from build123d import *

# Parameters (mm, degrees)
F0_W      = 79.172081314
F0_H      = 54.2475348338
F1_DEPTH  = 2
F2_W      = 79.172081314
F2_H      = 1.9382014871
F3_DEPTH  = 4
F4_W      = 52.3093333468
F4_H      = 4
F5_DEPTH  = 2.3
F6_W      = 76.872081314
F6_H      = 4
F7_DEPTH  = 2.1
F8_W      = 50.2093333468
F8_H      = 4
F9_DEPTH  = 2.4
F10_R     = 11.306687144
F11_DEPTH = 21
F12_R     = 9.8017826829
F13_DEPTH = 11
F14_R     = 8.8437005901
F15_DEPTH = 18


with BuildPart() as f1:
    # F0 (on Top) → F1 (new body)
    with BuildSketch(Plane.XY):
        with Locations((-27.7679827996, 36.830064375)):
            Rectangle(F0_W, F0_H)
    extrude(amount=F1_DEPTH)

    # F2 (on face) → F3 (join)
    with BuildSketch(Plane.XY.offset(2)):
        with Locations((-27.7679827996, 62.9847310483)):
            Rectangle(F2_W, F2_H)
    extrude(amount=F3_DEPTH)

    # F4 (on face) → F5 (join)
    with BuildSketch(Plane.YZ.offset(11.8180578575)):
        with Locations((35.8609636314, 4)):
            Rectangle(F4_W, F4_H)
    extrude(amount=-F5_DEPTH)

    # F6 (on face) → F7 (join)
    with BuildSketch(Plane.XZ.offset(-9.706296958)):
        with Locations((-28.9179827996, 4)):
            Rectangle(F6_W, F6_H)
    extrude(amount=-F7_DEPTH)

    # F8 (on face) → F9 (join)
    with BuildSketch(Plane(origin=(-67.3540234566, 0, 0), x_dir=(0, -1, 0), z_dir=(-1, 0, 0))):
        with Locations((-36.9109636314, 4)):
            Rectangle(F8_W, F8_H)
    extrude(amount=-F9_DEPTH)

    # F10 (on face) → F11 (join)
    with BuildSketch(Plane.XY.offset(2)):
        with Locations((-31.4333550632, 37.8074981272)):
            Circle(F10_R)
    extrude(amount=F11_DEPTH)

    # F12 (on face) → F13 (join)
    with BuildSketch(Plane.XY.offset(23)):
        with Locations((-31.4333550632, 37.8074981272)):
            Circle(F12_R)
    extrude(amount=-F13_DEPTH)

    # F14 (on face) → F15 (cut)
    with BuildSketch(Plane.XY.offset(23)):
        with Locations((-31.4333550632, 37.8074981272)):
            Circle(F14_R)
    extrude(amount=-F15_DEPTH, mode=Mode.SUBTRACT)


solid = f1.part
The model under review builds one solid part; all positions refer to its coordinate system, in mm. A direction names the side the tool comes from. Give positions to 0.01 mm unless a question says otherwise; leave off trailing zeros. Order: outer loops, then holes, each group sorted by start corner. A loop starts at its lowest first (then second) coordinate and runs counter-clockwise, first axis right, second up. Notation, with made-up numbers: M 38.5,-6 L 43.5,-6 A24 cw 43.5,11 Z; hole C -21,81 d4. An arc over 180 degrees is marked long. Answer in a Markdown table with one row per item. Add a question column.
1. To check wall thickness, follow line 1 along Y through (x, z) = (-35.5, 4.5); line 2 along X through (y, z) = (20, 4.5); line 3 along Z through (x, y) = (-25.5, 35.5). State the ranges of each line that lie inside material, in increasing order.
2. Add section D-D on x = -29. State the section outline as (y, z) points, plus the area to 3 significant figures.
3. Mouldability with a two-part tool opening along Y and no side actions: class faces 3 (the cylindrical face through (-25.35, 47.34, 12.35)), 4 (the flat face through (-28, 9.706, 3)), 5 (the flat face through (-28, 63, 6)), 6 (the flat face through (-64.954, 37, 4)) as released by +Y, released by -Y, zero draft, split by the parting line, or undercut.
4. Machinability: for faces 1 (the flat face through (11.818, 36, 3)), 2 (the flat face through (-28, 62.016, 4)), which of the approach directions +Z, -Z, +X, -X, +Y, -Y give a long, thin tool a straight path to every point of the face, cutting with its end or side? Answer none if there is none.
5. Add section B-B on x = 4. State the section outline as (y, z) points, plus the area to 3 significant figures.
6. Add section C-C on z = 16. State the section outline as (x, y) points.
7. For pin 1 Ø5 at (x, y) = (-25, 20.5) entering from +Z; pin 2 Ø3 at (x, z) = (-52.5, 9) entering from -Y; pin 3 Ø6 at (x, z) = (-20, 14) entering from +Y, all flat-tipped, find the tip position at first contact; note any pin that passes through.
8. Add section A-A on y = 56. State the section outline as (x, z) points, plus the area to 3 significant figures.
The answers:
| question | item | result |
|---|---|---|
| 1 | line 1 | 9.71 to 11.81, 27.26 to 48.36, 62.02 to 63.95 |
| 1 | line 2 | -67.35 to -64.95, 9.52 to 11.82 |
| 1 | line 3 | 0 to 5 |
| 2 | outline | M 9.71,0 L 63.95,0 L 63.95,6 L 62.02,6 L 62.02,2 L 48.85,2 L 48.85,23 L 46.31,23 L 46.31,5 L 29.31,5 L 29.31,23 L 26.77,23 L 26.77,2 L 11.81,2 L 11.81,6 L 9.71,6 Z |
| 2 | area | 282 mm2 |
| 3 | face 3 | undercut |
| 3 | face 4 | released by -Y |
| 3 | face 5 | zero draft |
| 3 | face 6 | undercut |
| 4 | face 1 | +Z, -Z, +X, +Y, -Y |
| 4 | face 2 | +Z |
| 5 | outline | M 9.71,0 L 63.95,0 L 63.95,6 L 62.02,6 L 62.02,2 L 11.81,2 L 11.81,6 L 9.71,6 Z |
| 5 | area | 125 mm2 |
| 6 | outline | C -31.43,37.81 d22.61; hole C -31.43,37.81 d17.69 |
| 7 | pin 1 | z = 2 |
| 7 | pin 2 | through |
| 7 | pin 3 | y = 45.34 |
| 8 | outline | M -67.35,0 L 11.82,0 L 11.82,6 L 9.52,6 L 9.52,2 L -64.95,2 L -64.95,6 L -67.35,6 Z |
| 8 | area | 177 mm2 |
